```python
from build123d import *

# Parameters (mm, degrees)
SKETCH1_W                                       = 203.2
SKETCH1_H                                       = 107.15625
BOSS_EXTRUDE1_DEPTH                             = 6.35
CSK_FOR_M2_FLAT_HEAD_MACHINE_SCREW1_D           = 2.4
CSK_FOR_M2_FLAT_HEAD_MACHINE_SCREW1_CSINK_D     = 4.4
CSK_FOR_M2_FLAT_HEAD_MACHINE_SCREW1_CSINK_ANGLE = 90
SKETCH4_W                                       = 4.943628295
SKETCH4_H                                       = 11.218233438
BOSS_EXTRUDE2_DEPTH                             = 1.27
SKETCH5_R                                       = 2.2
SKETCH5_W                                       = 33.85522898
SKETCH5_H                                       = 80.444626197
CUT_EXTRUDE1_DEPTH                              = 230.810844857


with BuildPart() as part:
    # Sketch1 → Boss-Extrude1 (new body)
    with BuildSketch(Plane(origin=(0, 0, 0), x_dir=(1, 0, 0), z_dir=(0, 1, 0))):
        with Locations((101.6, 53.578125)):
            Rectangle(SKETCH1_W, SKETCH1_H)
    extrude(amount=BOSS_EXTRUDE1_DEPTH)

    # CSK for M2 Flat Head Machine Screw1 (through all)
    with Locations(Plane(origin=(0, 6.35, 0), x_dir=(1, 0, 0), z_dir=(0, 1, 0))):
        with Locations((5.55625, 101.6), (1.201469153, 116.400099152), (1.201469153, 113.370035287), (29.36875, 101.6), (5.55625, 5.55625), (29.36875, 5.55625), (173.83125, 5.55625), (173.83125, 101.6), (197.64375, 101.6), (197.64375, 5.55625), (5.55625, 83.34375), (29.36875, 83.34375), (5.55625, 23.8125), (173.83125, 83.34375), (197.64375, 83.34375), (173.83125, 23.8125), (197.64375, 23.8125), (29.36875, 23.8125)):
            CounterSinkHole(CSK_FOR_M2_FLAT_HEAD_MACHINE_SCREW1_D / 2, CSK_FOR_M2_FLAT_HEAD_MACHINE_SCREW1_CSINK_D / 2, counter_sink_angle=CSK_FOR_M2_FLAT_HEAD_MACHINE_SCREW1_CSINK_ANGLE)

    # Sketch4 → Boss-Extrude2 (add)
    with BuildSketch(Plane(origin=(0, 6.35, 0), x_dir=(1, 0, 0), z_dir=(0, 1, 0))):
        with Locations((17.463249219, 14.029098644)):
            Rectangle(SKETCH4_W, SKETCH4_H)
    extrude(amount=BOSS_EXTRUDE2_DEPTH)

    # Sketch5 → Cut-Extrude1 (cut, through all)
    # profile 1 of 14: a face of its own
    with BuildSketch(Plane(origin=(0, 6.35, 0), x_dir=(1, 0, 0), z_dir=(0, 1, 0))):
        Polygon((203.2, 107.15625), (33.85522898, 107.15625), (33.85522898, 26.711623803), (33.85522898, 0), (203.2, 0), align=None)
        with Locations((173.83125, 5.55625)):
            Circle(SKETCH5_R, mode=Mode.SUBTRACT)
        with Locations((197.64375, 5.55625)):
            Circle(SKETCH5_R, mode=Mode.SUBTRACT)
        with Locations((173.83125, 23.8125)):
            Circle(SKETCH5_R, mode=Mode.SUBTRACT)
        with Locations((197.64375, 23.8125)):
            Circle(SKETCH5_R, mode=Mode.SUBTRACT)
        with Locations((173.83125, 83.34375)):
            Circle(SKETCH5_R, mode=Mode.SUBTRACT)
        with Locations((197.64375, 83.34375)):
            Circle(SKETCH5_R, mode=Mode.SUBTRACT)
        with Locations((173.83125, 101.6)):
            Circle(SKETCH5_R, mode=Mode.SUBTRACT)
        with Locations((197.64375, 101.6)):
            Circle(SKETCH5_R, mode=Mode.SUBTRACT)
    # profile 2 of 14: a face of its own
    with BuildSketch(Plane(origin=(0, 6.35, 0), x_dir=(1, 0, 0), z_dir=(0, 1, 0))):
        with Locations((16.92761449, 66.933936902)):
            Rectangle(SKETCH5_W, SKETCH5_H)
        with Locations((5.55625, 83.34375)):
            Circle(SKETCH5_R, mode=Mode.SUBTRACT)
        with Locations((29.36875, 83.34375)):
            Circle(SKETCH5_R, mode=Mode.SUBTRACT)
        with Locations((5.55625, 101.6)):
            Circle(SKETCH5_R, mode=Mode.SUBTRACT)
        with Locations((29.36875, 101.6)):
            Circle(SKETCH5_R, mode=Mode.SUBTRACT)
    # profile 3 of 14: a face of its own
    with BuildSketch(Plane(origin=(0, 6.35, 0), x_dir=(1, 0, 0), z_dir=(0, 1, 0))):
        with Locations((5.55625, 83.34375)):
            Circle(SKETCH5_R)
    # profile 4 of 14: a face of its own
    with BuildSketch(Plane(origin=(0, 6.35, 0), x_dir=(1, 0, 0), z_dir=(0, 1, 0))):
        with Locations((5.55625, 101.6)):
            Circle(SKETCH5_R)
    # profile 5 of 14: a face of its own
    with BuildSketch(Plane(origin=(0, 6.35, 0), x_dir=(1, 0, 0), z_dir=(0, 1, 0))):
        with Locations((29.36875, 101.6)):
            Circle(SKETCH5_R)
    # profile 6 of 14: a face of its own
    with BuildSketch(Plane(origin=(0, 6.35, 0), x_dir=(1, 0, 0), z_dir=(0, 1, 0))):
        with Locations((29.36875, 83.34375)):
            Circle(SKETCH5_R)
    # profile 7 of 14: a face of its own
    with BuildSketch(Plane(origin=(0, 6.35, 0), x_dir=(1, 0, 0), z_dir=(0, 1, 0))):
        with Locations((173.83125, 101.6)):
            Circle(SKETCH5_R)
    # profile 8 of 14: a face of its own
    with BuildSketch(Plane(origin=(0, 6.35, 0), x_dir=(1, 0, 0), z_dir=(0, 1, 0))):
        with Locations((197.64375, 101.6)):
            Circle(SKETCH5_R)
    # profile 9 of 14: a face of its own
    with BuildSketch(Plane(origin=(0, 6.35, 0), x_dir=(1, 0, 0), z_dir=(0, 1, 0))):
        with Locations((173.83125, 83.34375)):
            Circle(SKETCH5_R)
    # profile 10 of 14: a face of its own
    with BuildSketch(Plane(origin=(0, 6.35, 0), x_dir=(1, 0, 0), z_dir=(0, 1, 0))):
        with Locations((197.64375, 83.34375)):
            Circle(SKETCH5_R)
    # profile 11 of 14: a face of its own
    with BuildSketch(Plane(origin=(0, 6.35, 0), x_dir=(1, 0, 0), z_dir=(0, 1, 0))):
        with Locations((173.83125, 23.8125)):
            Circle(SKETCH5_R)
    # profile 12 of 14: a face of its own
    with BuildSketch(Plane(origin=(0, 6.35, 0), x_dir=(1, 0, 0), z_dir=(0, 1, 0))):
        with Locations((197.64375, 23.8125)):
            Circle(SKETCH5_R)
    # profile 13 of 14: a face of its own
    with BuildSketch(Plane(origin=(0, 6.35, 0), x_dir=(1, 0, 0), z_dir=(0, 1, 0))):
        with Locations((173.83125, 5.55625)):
            Circle(SKETCH5_R)
    # profile 14 of 14: a face of its own
    with BuildSketch(Plane(origin=(0, 6.35, 0), x_dir=(1, 0, 0), z_dir=(0, 1, 0))):
        with Locations((197.64375, 5.55625)):
            Circle(SKETCH5_R)
    extrude(amount=-CUT_EXTRUDE1_DEPTH, mode=Mode.SUBTRACT)


solid = part.part
```
Work out the finished part from the listing and answer in its coordinate system (mm). A direction names the side the tool comes from. Round coordinates to 2 decimals unless told otherwise and drop trailing zeros. Loops run counter-clockwise (first coordinate to the right, second up) from the corner with the lowest first, then second, coordinate; pieces in that order, holes last. Notation, with made-up numbers: M -21,75 L 16,75 A34 ccw 16,111 Z; hole C -10,5 d1. An arc over 180 degrees is marked long. Use CSV: the item, a comma, the result in double quotes.
Q1. Section A-A, the plane z = -18 is taken. Determine the outline of the cut face in (x, y).
Determined:
outline,"M 0,0 L 33.86,0 L 33.86,6.35 L 19.94,6.35 L 19.94,7.62 L 14.99,7.62 L 14.99,6.35 L 0,6.35 Z"
Q2. Consider L1, parallel to Z at x = 29.5, y = 5; L2, parallel to Z at x = 30, y = 2; L3, parallel to X at y = 6.25, z = -25. Determine where each line is inside the solid, lowest interval first.
Determined:
L1,"-26.71 to -25.01, -22.62 to -6.75, -4.36 to 0"
L2,"-26.71 to -24.83, -22.79 to -6.58, -4.54 to 0"
L3,"0 to 3.82, 7.29 to 27.64, 31.1 to 33.86"
Q3. A tool of negligible diameter and unlimited length cuts with its end or side. For faces 1 (the flat face through (19.935, 7, -14)), 2 (the flat face through (14.991, 7, -14)), 3 (the flat face through (17, 7.62, -14)), from which of +Z, -Z, +X, -X, +Y, -Y can it reach the whole face along a straight path? Write none if from no direction.
Determined:
face 1,"+Z, -Z, +X, +Y"
face 2,"+Z, -Z, -X, +Y"
face 3,"+Z, -Z, +X, -X, +Y"
Q4. Each of these flat-tipped pins is pushed along its axis until it touches: pin 1 (1.4 mm diameter, centred on x = 5.56, z = -23.81, fed in from -Y); pin 2 (1 mm diameter, centred on y = 7, z = -15.5, fed in from -X); pin 3 (3 mm diameter, centred on x = 5.56, z = -5.56, fed in from +Y). Where does it stop, or does it pass through?
Determined:
pin 1,"through"
pin 2,"x = 14.99"
pin 3,"y = 5.66"
Q5. Section B-B, the plane y = 1.5 is taken. Determine the outline of the cut face in (x, z).
Determined:
outline,"M 0,-26.71 L 33.86,-26.71 L 33.86,0 L 0,0 Z; hole C 5.56,-23.81 d2.4; hole C 5.56,-5.56 d2.4; hole C 29.37,-23.81 d2.4; hole C 29.37,-5.56 d2.4"
Q6. Section C-C, the plane x = 16.5 is taken. Determine the outline of the cut face in (y, z), then the cut area to 3 significant figures.
Determined:
outline,"M 0,-26.71 L 6.35,-26.71 L 6.35,-19.64 L 7.62,-19.64 L 7.62,-8.42 L 6.35,-8.42 L 6.35,0 L 0,0 Z"
area,"184 mm2"
Q7. Section D-D, the plane y = 7.25 is taken. Determine the outline of the cut face in (x, z), then the cut area to 3 significant figures.
Determined:
outline,"M 14.99,-19.64 L 19.94,-19.64 L 19.94,-8.42 L 14.99,-8.42 Z"
area,"55.5 mm2"
Q8. The mould has two halves that part along X. Classify faces 4 (the flat face through (33.855, 3, -14)), 5 (the cylindrical face through (28.815, 2.638, -22.748)), 6 (the flat face through (17, 7, -8.42)): pulls with the +X half, pulls with the -X half, needs draft (parallel to the pull), parting line crosses it, or undercut.
Determined:
face 4,"pulls with the +X half"
face 5,"undercut"
face 6,"needs draft"
